```python
from build123d import *

# Parameters (mm, degrees)
SKETCH1_W           = 100
SKETCH1_H           = 100
BOSS_EXTRUDE1_DEPTH = 135
FILLET1_R           = 20
SHELL1_T            = 1.5


with BuildPart() as part:
    # Sketch1 → Boss-Extrude1 (new body)
    with BuildSketch(Plane(origin=(0, 0, 0), x_dir=(1, 0, 0), z_dir=(0, 1, 0))):
        Rectangle(SKETCH1_W, SKETCH1_H)
    extrude(amount=BOSS_EXTRUDE1_DEPTH)

    # Fillet1
    fillet1_edges = [part.edges().sort_by_distance(p)[0] for p in [
        (50, 135, 0),
        (0, 135, -50),
        (-50, 135, 0),
        (0, 0, -50),
        (50, 0, 0),
        (0, 0, 50),
        (-50, 0, 0),
        (-50, 67.5, -50),
        (50, 67.5, -50),
        (50, 67.5, 50),
        (-50, 67.5, 50),
        (0, 135, 50),
    ]]
    fillet(fillet1_edges, radius=FILLET1_R)

    # Shell1 (no face opened: a closed hollow body)
    add(offset(amount=-SHELL1_T, mode=Mode.PRIVATE), mode=Mode.SUBTRACT)


solid = part.part
```
The listing builds one solid part. Answer for the finished solid, in the listing's coordinates (mm). A direction names the side the tool comes from. Round coordinates to 2 decimals unless told otherwise and drop trailing zeros. Loops run counter-clockwise (first coordinate to the right, second up) from the corner with the lowest first, then second, coordinate; pieces in that order, holes last.
Q1. Section A-A, the plane x = -21 is taken. Determine the outline of the cut face in (y, z).
Q2. Find the intervals of material crossed by line 1 (X direction, y = 66, z = -12.5); line 2 (Y direction, x = 28, z = -27.5), in increasing order.
Q3. Given pin 1 Ø1.5 at (x, z) = (38.5, -23) entering from +Y; pin 2 Ø3 at (y, z) = (61.5, -38) entering from +X; pin 3 Ø6 at (x, y) = (-36, 17.5) entering from -Z, each flat-ended and moving along its own axis, determine where each tip first touches the part or whether it passes through.
Q4. For a pull along Z with two mould halves and no side action, classify faces 3 (the face through (-44.297, 68.165, -43.986)), 4 (the face through (44.297, 128.986, -0.42)), 5 (the face through (0, 67, -48.5)) as released by +Z, released by -Z, zero draft, split by the parting line, or undercut.
Q5. Section B-B, the plane y = 48 is taken. Determine the outline of the cut face in (x, z), then the cut area to 3 significant figures.
Q6. Which of the six approach directions +Z, -Z, +X, -X, +Y, -Y give full straight-line access (tool end or side, diameter ignored) to faces 1 (the face through (42.94, 68.16, 43.22)), 2 (the face through (-44.297, 128.986, -0.42))?
Completed:
1. outline: (0, -30) arc R20 ccw to (20, -50) - (115, -50) arc R20 ccw to (135, -30) - (135, 30) arc R20 ccw to (115, 50) - (20, 50) arc R20 ccw to (0, 30) - close; hole (1.5, -30) arc R18.5 ccw to (20, -48.5) - (115, -48.5) arc R18.5 ccw to (133.5, -30) - (133.5, 30) arc R18.5 ccw to (115, 48.5) - (20, 48.5) arc R18.5 ccw to (1.5, 30) - close
2. line 1: x = -50 to -48.5, 48.5 to 50
2. line 2: y = 0 to 1.5, 133.5 to 135
3. pin 1: stops at y = 133.44
3. pin 2: stops at x = 48.91
3. pin 3: stops at z = -49.69
4. face 3: released by -Z
4. face 4: zero draft
4. face 5: undercut
5. outline: (-50, -30) arc R20 ccw to (-30, -50) - (30, -50) arc R20 ccw to (50, -30) - (50, 30) arc R20 ccw to (30, 50) - (-30, 50) arc R20 ccw to (-50, 30) - close; hole (-48.5, -30) arc R18.5 ccw to (-30, -48.5) - (30, -48.5) arc R18.5 ccw to (48.5, -30) - (48.5, 30) arc R18.5 ccw to (30, 48.5) - (-30, 48.5) arc R18.5 ccw to (-48.5, 30) - close
5. area: 541 mm2
6. face 1: none
6. face 2: +Z, -Z, -X, +Y
